Design review of the part built by this model. Coordinates are the model's own, in mm. Coordinates: 2 decimals unless noted, no trailing zeros. Write each loop counter-clockwise with the first axis right and the second up, starting at its lowest first coordinate (ties: lowest second). Pieces come first, ordered by that corner, then holes. Notation, with made-up numbers: (21, 9) - (66, 9) arc R16 ccw to (66, 39) - close; hole circle Ø1 at (-20, -30.75). An arc over 180 degrees is marked (long way). Answer as CSV lines item,"result". Start each with the question number.
Q1. We need section B-B (x = -139.7). Write out the cut boundary in (y, z) (3 decimals).
Q2. For line 1 along X through (y, z) = (0.55, -139.5); line 2 along X through (y, z) = (0.85, -12.7) (3 decimals); line 3 along Z through (x, y) = (-139.7, 0.85) (3 decimals), list the stretches that pass through material, from the lowest coordinate up. Write a range as [from, to].
Q3. We need section A-A (z = -139.7). Write out the cut boundary in (x, y) (3 decimals), plus the area to 3 significant figures.
Q4. We need section C-C (z = -12.7). Write out the cut boundary in (x, y) (3 decimals), plus the area to 3 significant figures.
Q5. Mouldability with a two-part tool opening along X and no side actions: class faces 1 (the face through (-85.8, 1.57, -140.39)), 2 (the face through (-75, 0, -75)) as pulls with the +X half, pulls with the -X half, needs draft (parallel to the pull), parting line crosses it, or undercut.
Autodesk Inventor part; units mm, degrees
ref_plane "YZ Plane" through (0, 0, 0) normal (1, 0, 0) x (0, 1, 0)
ref_plane "XZ Plane" through (0, 0, 0) normal (0, 1, 0) x (-1, 0, 0)
ref_plane "XY Plane" through (0, 0, 0) normal (0, 0, 1) x (1, 0, 0)
sketch "Sketch1" plane through (0, 0, 0) normal (0, 1, 0) x (-1, 0, 0)
  line L0 (0, 0) -> (152.4, 0)
  line L1 (152.4, 0) -> (152.4, -152.4)
  line L2 (152.4, -152.4) -> (0, -152.4)
  line L3 (0, -152.4) -> (0, 0)
  dimension "d0" = 152.4
  dimension "d1" = 152.4
extrude "Extrusion1" add sketch "Sketch1" along normal blind 3.175
sketch "Sketch2" plane through (0, 3.175, 0) normal (0, 1, 0) x (1, 0, 0)
  line L0 (-152.4, 0) -> (0, 0)
  line L1 (0, 0) -> (0, 152.4)
  line L2 (0, 152.4) -> (-152.4, 152.4)
  line L3 (-152.4, 152.4) -> (-152.4, 0)
  point P0 (-139.7, 12.7)
  point P1 (-63.5, 12.7)
  point P2 (-12.7, 12.7)
  point P3 (-12.7, 139.7)
  point P4 (-63.5, 139.7)
  point P5 (-139.7, 139.7)
  dimension "d4" = 12.7
  dimension "d5" = 12.7
  dimension "d6" = 12.7
  dimension "d7" = 12.7
  dimension "d8" = 12.7
  dimension "d9" = 12.7
  dimension "d10" = 12.7
  dimension "d11" = 63.5
  dimension "d12" = 12.7
  dimension "d13" = 12.7
  dimension "d14" = 12.7
  dimension "d15" = 63.5
hole "Hole1" at (-139.7, 3.175, -12.7) at (-63.5, 3.175, -12.7) at (-12.7, 3.175, -12.7) at (-12.7, 3.175, -139.7) at (-63.5, 3.175, -139.7) at (-139.7, 3.175, -139.7) direction (0, -1, 0) diameter 6.35 end through all
sketch "Sketch3" plane through (0, 3.175, 0) normal (0, 1, 0) x (1, 0, 0)
  circle A0 centre (-139.7, 139.7) radius 3.175
  line L0 (0, 152.4) -> (-152.4, 152.4)
  point P0 (-88.9, 139.7)
  dimension "d23" = 12.7
  dimension "d24" = 50.8
hole "Hole2" at (-88.9, 3.175, -139.7) direction (0, -1, 0) diameter 6.35 end through all
properties part number "pickup arm plate" material "Aluminum 6061"
Results list:
1,outline,"(0, -152.4) - (3.175, -152.4) - (3.175, -142.875) - (0, -142.875) - close; (0, -136.525) - (3.175, -136.525) - (3.175, -15.875) - (0, -15.875) - close; (0, -9.525) - (3.175, -9.525) - (3.175, 0) - (0, 0) - close"
2,line 1,"x = [-152.4, -142.87], [-136.53, -92.07], [-85.73, -66.67], [-60.33, -15.87], [-9.53, 0]"
2,line 2,"x = [-152.4, -142.875], [-136.525, -66.675], [-60.325, -15.875], [-9.525, 0]"
2,line 3,"z = [-152.4, -142.875], [-136.525, -15.875], [-9.525, 0]"
3,outline,"(-152.4, 0) - (-142.875, 0) - (-142.875, 3.175) - (-152.4, 3.175) - close; (-136.525, 0) - (-92.075, 0) - (-92.075, 3.175) - (-136.525, 3.175) - close; (-85.725, 0) - (-66.675, 0) - (-66.675, 3.175) - (-85.725, 3.175) - close; (-60.325, 0) - (-15.875, 0) - (-15.875, 3.175) - (-60.325, 3.175) - close; (-9.525, 0) - (0, 0) - (0, 3.175) - (-9.525, 3.175) - close"
3,area,"403 mm2"
4,outline,"(-152.4, 0) - (-142.875, 0) - (-142.875, 3.175) - (-152.4, 3.175) - close; (-136.525, 0) - (-66.675, 0) - (-66.675, 3.175) - (-136.525, 3.175) - close; (-60.325, 0) - (-15.875, 0) - (-15.875, 3.175) - (-60.325, 3.175) - close; (-9.525, 0) - (0, 0) - (0, 3.175) - (-9.525, 3.175) - close"
4,area,"423 mm2"
5,face 1,"undercut"
5,face 2,"needs draft"
